from build123d import *

# Parameters (mm, degrees)
SKETCH038_W          = 55
SKETCH038_H          = 29.5
PAD009_DEPTH         = 4.5
THICKNESS003_T       = 1.5
SKETCH039_W          = 55
SKETCH039_H          = 29.5
SKETCH039_W_2        = 53
SKETCH039_H_2        = 27.5
PAD010_DEPTH         = 4.5
PAD010_DEPTH_BACK    = 3
SKETCH040_W          = 15.180022
SKETCH040_H          = 15.677626
POCKET024_DEPTH      = 29.001
POCKET024_DEPTH_BACK = 29.001
SKETCH043_W          = 20
SKETCH043_H          = 27
SKETCH043_W_2        = 29.5
SKETCH043_H_2        = 27.5
POCKET026_DEPTH      = 1.1
SKETCH042_W          = 12
SKETCH042_H          = 24
POCKET029_DEPTH      = 6.001
POCKET030_DEPTH      = 14.75
CHAMFER006_SIZE      = 0.75


with BuildPart() as part:
    # Sketch038 → Pad009 (new body)
    with BuildSketch(Plane.XY):
        Rectangle(SKETCH038_W, SKETCH038_H)
    extrude(amount=PAD009_DEPTH)

    # Thickness003
    thickness003_openings = [part.faces().sort_by_distance(p)[0] for p in [
        (0, 0, 0),
    ]]
    offset(amount=THICKNESS003_T, openings=thickness003_openings)

    # Sketch039 → Pad010 (join, two sides)
    with BuildSketch(Plane.XY) as pad010_sk:
        Rectangle(SKETCH039_W, SKETCH039_H)
        Rectangle(SKETCH039_W_2, SKETCH039_H_2, mode=Mode.SUBTRACT)
    extrude(amount=PAD010_DEPTH)
    extrude(pad010_sk.sketch, amount=-PAD010_DEPTH_BACK)

    # Sketch040 → Pocket024 (cut, two sides)
    with BuildSketch(Plane.YZ) as pocket024_sk:
        with Locations((0, -7.838813)):
            Rectangle(SKETCH040_W, SKETCH040_H)
    extrude(amount=POCKET024_DEPTH, mode=Mode.SUBTRACT)
    extrude(pocket024_sk.sketch, amount=-POCKET024_DEPTH_BACK, mode=Mode.SUBTRACT)

    # Sketch043 → Pocket026 (cut)
    with BuildSketch(Plane.XY.offset(4.5)):
        with Locations((13.75, 0)):
            Rectangle(SKETCH043_W, SKETCH043_H)
        with Locations((-12.75, 0)):
            Rectangle(SKETCH043_W_2, SKETCH043_H_2)
    extrude(amount=POCKET026_DEPTH, mode=Mode.SUBTRACT)

    # Sketch042 → Pocket029 (cut, through all)
    with BuildSketch(Plane.XY):
        with Locations((16.5, 0)):
            Rectangle(SKETCH042_W, SKETCH042_H)
    extrude(amount=POCKET029_DEPTH, mode=Mode.SUBTRACT)

    # Sketch051 → Pocket030 (cut, symmetric)
    with BuildSketch(Plane.XZ):
        Polygon((23, 3.25), (23, 4.25), (7.978224, 4.25), (0.497934, 2.75), (-22, 2.75), (-22, 1.75), (0.696514, 1.75), (8.176805, 3.25), align=None)
    extrude(amount=POCKET030_DEPTH, both=True, mode=Mode.SUBTRACT)

    # Chamfer006
    chamfer006_edges = [part.edges().sort_by_distance(p)[0] for p in [
        (0.497934, -14.25, 2.75),
        (-22, 14.75, 2.25),
        (-10.751033, 14.75, 2.75),
        (4.238079, 14.75, 3.5),
        (7.978224, -14.25, 4.25),
        (15.489112, -14.75, 4.25),
    ]]
    chamfer(chamfer006_edges, length=CHAMFER006_SIZE)


with BuildPart() as part_1:
    # Body004 placement: moved
    add(part.part.moved(Location((0, 0, 13.5))))


solid = part_1.part
For this review, take the finished solid that the model builds, in its own axes (mm). A direction names the side the tool comes from. Coordinates: 2 decimals unless noted, no trailing zeros. Order: outer loops, then holes, each group sorted by start corner. A loop starts at its lowest first (then second) coordinate and runs counter-clockwise, first axis right, second up. Notation, with made-up numbers: (-18.75, 7.5) -> (34.25, 7.5) arc R33 ccw to (34.25, 44.5) -> close; hole circle Ø10 at (26, -14.75). An arc over 180 degrees is marked (long way). Return JSON: item names as keys, results as strings.
1. The part is to be moulded in two halves that separate along Z. For faces 6 (the flat face through (4.38, -14.26, 15.99)), 7 (the flat face through (-6, 0, 19.5)), 8 (the flat face through (-29, 0, 16)), 9 (the flat face through (9, 14.75, 17)), say which applies: +Z half, -Z half, draft (parallel to the pull), parting line (faces both ways), or undercut.
Answer block:
{"face 6": "undercut", "face 7": "+Z half", "face 8": "draft", "face 9": "undercut"}
2. For line 1 (Y direction, x = -18, z = 15); line 2 (Y direction, x = -9.5, z = 11.5); line 3 (X direction, y = 7, z = 18.75), list the stretches that pass through material, from the lowest coordinate up. Write a range as from..to.
Answer block:
{"line 1": "-16.25..-13.75, 13.75..16.25", "line 2": "-14.75..-13.75, 13.75..14.75", "line 3": "-28.8..-27.5, 2..3.75, 23.75..28.8"}
3. For pin 1 Ø1.5 at (y, z) = (10, 12.5) entering from -X; pin 2 Ø0.8 at (x, z) = (-27, 12.5) entering from -Y; pin 3 Ø0.6 at (y, z) = (3.5, 18.5) entering from +X; pin 4 Ø1.2 at (x, z) = (13.5, 18.5) entering from +Y, all flat-tipped, find the tip position at first contact; note any pin that passes through.
Answer block:
{"pin 1": "x = -27.5", "pin 2": "y = -14.75", "pin 3": "x = 28.99", "pin 4": "y = 16.25"}
4. We need section D-D on x = -15. Write out the cut boundary in (y, z).
Answer block:
{"outline": "(-16.25, 13.5) -> (-14.75, 13.5) -> (-14.75, 10.5) -> (-13.75, 10.5) -> (-13.75, 15.25) -> (-14.75, 15.25) -> (-14.75, 16.25) -> (-13.75, 16.25) -> (-13.75, 19.1) -> (13.75, 19.1) -> (13.75, 16.25) -> (14, 16.25) -> (14.75, 15.5) -> (14.75, 15.25) -> (13.75, 15.25) -> (13.75, 10.5) -> (14.75, 10.5) -> (14.75, 13.5) -> (16.25, 13.5) -> (16.25, 18) arc R1.5 ccw to (14.75, 19.5) -> (-14.75, 19.5) arc R1.5 ccw to (-16.25, 18) -> close"}
5. Machinability: for faces 1 (the flat face through (27.5, 11, 12)), 2 (the flat face through (-5, -14.75, 16)), 3 (the flat face through (24, 0, 18)), 4 (the flat face through (0, -14.75, 12)), 5 (the cylindrical face through (-28.57, 0.21, 19.05)), which of the approach directions +Z, -Z, +X, -X, +Y, -Y give a long, thin tool a straight path to every point of the face, cutting with its end or side? Answer none if there is none.
Answer block:
{"face 1": "-Z, +X, +Y, -Y", "face 2": "none", "face 3": "-Z", "face 4": "-Z, +X, -X, -Y", "face 5": "+Z, -X, +Y, -Y"}
6. We need section B-B on y = -2.5. Write out the cut boundary in (x, z).
Answer block:
{"outline": "(-29, 13.5) -> (-26.5, 13.5) -> (-26.5, 18) -> (-27.5, 18) -> (-27.5, 19.1) -> (2, 19.1) -> (2, 18) -> (3.75, 18) -> (3.75, 19.1) -> (10.5, 19.1) -> (10.5, 19.5) -> (-27.5, 19.5) arc R1.5 ccw to (-29, 18) -> close; (22.5, 19.1) -> (23.75, 19.1) -> (23.75, 18) -> (26.5, 18) -> (26.5, 13.5) -> (29, 13.5) -> (29, 18) arc R1.5 ccw to (27.5, 19.5) -> (22.5, 19.5) -> close"}
7. We need section A-A on z = 12.75. Write out the cut boundary in (x, y), and give its area (3 significant figures).
Answer block:
{"outline": "(-27.5, -14.75) -> (27.5, -14.75) -> (27.5, -7.59) -> (26.5, -7.59) -> (26.5, -13.75) -> (-26.5, -13.75) -> (-26.5, -7.59) -> (-27.5, -7.59) -> close; (-27.5, 7.59) -> (-26.5, 7.59) -> (-26.5, 13.75) -> (26.5, 13.75) -> (26.5, 7.59) -> (27.5, 7.59) -> (27.5, 14.75) -> (-27.5, 14.75) -> close", "area": "135 mm²"}
